from build123d import *

# Parameters (mm, degrees)
BOSS_EXTRUDE1_DEPTH = 3


with BuildPart() as part:
    # Sketch1 → Boss-Extrude1 (new body)
    with BuildSketch(Plane(origin=(0, 3.6, 0), x_dir=(1, 0, 0), z_dir=(0, 1, 0))):
        with BuildLine():
            Line((-8.6, 7), (-8.6, 5.6))
            Line((-8.6, 5.6), (-10.613199329, 5.6))
            ThreePointArc((-10.613199329, 5.6), (-11.866912034, -1.782245428), (-8.5, -8.470537173))
            Line((-8.5, -8.470537173), (-8.5, -4))
            ThreePointArc((-8.5, -4), (0, 4.5), (8.5, -4))
            Line((8.5, -4), (8.5, -8.470537173))
            ThreePointArc((8.5, -8.470537173), (11.632283064, -2.947879019), (11.508257905, 3.4))
            Line((11.508257905, 3.4), (9.5, 3.4))
            Line((9.5, 3.4), (9.5, 4.8))
            Line((9.5, 4.8), (10.998181668, 4.8))
            ThreePointArc((10.998181668, 4.8), (6.985647075, 9.757086397), (1, 11.958260743))
            Line((1, 11.958260743), (1, 10.5))
            Line((1, 10.5), (0.4, 10.5))
            Line((0.4, 10.5), (-0.4, 10.5))
            Line((-0.4, 10.5), (-0.4, 11.99333148))
            ThreePointArc((-0.4, 11.99333148), (-5.654440617, 10.584295031), (-9.746794345, 7))
            Line((-9.746794345, 7), (-8.6, 7))
        make_face()
        with BuildLine():
            Line((0.4, 11.99333148), (0.4, 10.5))
            Line((0.4, 10.5), (1, 10.5))
            Line((1, 10.5), (1, 11.958260743))
            ThreePointArc((1, 11.958260743), (0.700219601, 11.979553101), (0.4, 11.99333148))
        make_face()
    extrude(amount=BOSS_EXTRUDE1_DEPTH)


solid = part.part
Design review of the part built by this model. Coordinates are the model's own, in mm. A direction names the side the tool comes from. Round coordinates to 2 decimals unless told otherwise and drop trailing zeros. Write each loop counter-clockwise with the first axis right and the second up, starting at its lowest first coordinate (ties: lowest second). Pieces come first, ordered by that corner, then holes.
Item 1: For faces 5 (the flat face through (-9, 5, -7)), 6 (the flat face through (0.4, 5, -11)), 7 (the flat face through (11, 5, -3.4)), list the 3-axis set-ups (+Z, -Z, +X, -X, +Y, -Y) from which the entire face can be reached by the end or side of a thin tool; tool diameter is ignored.
Item 2: Consider section D-D on z = 6.5. Give the boundary of the cut face in (x, y), and give its area (3 significant figures).
Item 3: Consider section A-A on z = -1.75. Give the boundary of the cut face in (x, y), and give its area (3 significant figures).
Item 4: Draft analysis for pull direction X (two halves, no side actions). For faces 1 (the flat face through (9.5, 5, -4)), 2 (the flat face through (-0.4, 5, -11)), 3 (the flat face through (8.5, 5, 6)), 4 (the cylindrical face through (-5.59, 5.08, -10.62)), state which applies: released by +X, released by -X, zero draft, split by the parting line, or undercut.
Item 5: Consider section C-C on x = 0. Give the boundary of the cut face in (y, z), and give its area (3 significant figures).
Item 6: Wall thickness on L1, parallel to X at y = 4.45, z = 5.75; L2, parallel to X at y = 4.2, z = 5.5; L3, parallel to Z at x = 0, y = 5.8: over which ranges is each line inside the solid? List them lowest first.
Item 7: For pin 1 Ø0.9 at (x, y) = (-9, 5) entering from +Z; pin 2 Ø3 at (x, z) = (0.5, -1.5) entering from -Y; pin 3 Ø0.7 at (y, z) = (4.5, -11) entering from +X; pin 4 Ø1.1 at (y, z) = (5.5, -4) entering from +X, all flat-tipped, find the tip position at first contact; note any pin that passes through.
Item 8: Consider section B-B on y = 4.55. Give the boundary of the cut face in (x, z), and give its area (3 significant figures).
Check values:
1. face 5: -X, +Y, -Y
1. face 6: -Z, +Y, -Y
1. face 7: +X, +Y, -Y
2. outline: (-10.09, 3.6) - (-8.5, 3.6) - (-8.5, 6.6) - (-10.09, 6.6) - close; (8.5, 3.6) - (10.09, 3.6) - (10.09, 6.6) - (8.5, 6.6) - close
2. area: 9.52 mm2
3. outline: (-11.87, 3.6) - (-6.26, 3.6) - (-6.26, 6.6) - (-11.87, 6.6) - close; (6.26, 3.6) - (11.87, 3.6) - (11.87, 6.6) - (6.26, 6.6) - close
3. area: 33.7 mm2
4. face 1: released by +X
4. face 2: undercut
4. face 3: undercut
4. face 4: released by -X
5. outline: (3.6, -10.5) - (6.6, -10.5) - (6.6, -4.5) - (3.6, -4.5) - close
5. area: 18.0 mm2
6. L1: x = -10.53 to -8.5, 8.5 to 10.53
6. L2: x = -10.67 to -8.5, 8.5 to 10.67
6. L3: z = -10.5 to -4.5
7. pin 1: stops at z = 8.42
7. pin 2: passes through
7. pin 3: stops at x = 5.53
7. pin 4: stops at x = 9.5
8. outline: (-10.61, -5.6) - (-8.6, -5.6) - (-8.6, -7) - (-9.75, -7) arc R12 ccw to (-0.4, -11.99) - (-0.4, -10.5) - (0.4, -10.5) - (0.4, -11.99) arc R12 ccw to (11, -4.8) - (9.5, -4.8) - (9.5, -3.4) - (11.51, -3.4) arc R12 ccw to (8.5, 8.47) - (8.5, 4) arc R8.5 cw to (-8.5, 4) - (-8.5, 8.47) arc R12 ccw to start
8. area: 216 mm2
